from build123d import *

# Parameters (mm, degrees)
BOSS_EXTRUDE1_DEPTH = 1


with BuildPart() as part:
    # Sketch1 → Boss-Extrude1 (new body)
    with BuildSketch(Plane(origin=(0, 0, 0), x_dir=(1, 0, 0), z_dir=(0, 1, 0))):
        with BuildLine():
            Line((-12.25, -13.3), (-12.25, -15))
            Line((-12.25, -15), (12.25, -15))
            Line((12.25, -15), (12.25, -13.3))
            ThreePointArc((12.25, -13.3), (11.50753788, -11.50753788), (13.3, -12.25))
            Line((13.3, -12.25), (15, -12.25))
            Line((15, -12.25), (15, 12.25))
            Line((15, 12.25), (13.3, 12.25))
            ThreePointArc((13.3, 12.25), (11.50753788, 11.50753788), (12.25, 13.3))
            Line((12.25, 13.3), (12.25, 15))
            Line((12.25, 15), (-12.25, 15))
            Line((-12.25, 15), (-12.25, 13.3))
            ThreePointArc((-12.25, 13.3), (-11.50753788, 12.99246212), (-11.2, 12.25))
            ThreePointArc((-11.2, 12.25), (-12.25, 11.2), (-13.3, 12.25))
            Line((-13.3, 12.25), (-15, 12.25))
            Line((-15, 12.25), (-15, -12.25))
            Line((-15, -12.25), (-13.3, -12.25))
            ThreePointArc((-13.3, -12.25), (-12.25, -11.2), (-11.2, -12.25))
            ThreePointArc((-11.2, -12.25), (-11.50753788, -12.99246212), (-12.25, -13.3))
        make_face()
        with BuildLine():
            Line((-15, 12.5), (-15, 12.25))
            Line((-15, 12.25), (-13.3, 12.25))
            ThreePointArc((-13.3, 12.25), (-12.99246212, 12.99246212), (-12.25, 13.3))
            Line((-12.25, 13.3), (-12.25, 15))
            Line((-12.25, 15), (-12.5, 15))
            ThreePointArc((-12.5, 15), (-14.267766953, 14.267766953), (-15, 12.5))
        make_face()
        with BuildLine():
            Line((13.3, 12.25), (15, 12.25))
            Line((15, 12.25), (15, 12.5))
            ThreePointArc((15, 12.5), (14.267766953, 14.267766953), (12.5, 15))
            Line((12.5, 15), (12.25, 15))
            Line((12.25, 15), (12.25, 13.3))
            ThreePointArc((12.25, 13.3), (12.99246212, 12.99246212), (13.3, 12.25))
        make_face()
        with BuildLine():
            Line((12.25, -13.3), (12.25, -15))
            Line((12.25, -15), (12.5, -15))
            ThreePointArc((12.5, -15), (14.267766953, -14.267766953), (15, -12.5))
            Line((15, -12.5), (15, -12.25))
            Line((15, -12.25), (13.3, -12.25))
            ThreePointArc((13.3, -12.25), (12.99246212, -12.99246212), (12.25, -13.3))
        make_face()
        with BuildLine():
            ThreePointArc((-15, -12.5), (-14.267766953, -14.267766953), (-12.5, -15))
            Line((-12.5, -15), (-12.25, -15))
            Line((-12.25, -15), (-12.25, -13.3))
            ThreePointArc((-12.25, -13.3), (-12.99246212, -12.99246212), (-13.3, -12.25))
            Line((-13.3, -12.25), (-15, -12.25))
            Line((-15, -12.25), (-15, -12.5))
        make_face()
    extrude(amount=BOSS_EXTRUDE1_DEPTH)


solid = part.part
Could you check a few things on this model? Use its own coordinates, in mm. Round coordinates to 2 decimals unless told otherwise and drop trailing zeros. Loops run counter-clockwise (first coordinate to the right, second up) from the corner with the lowest first, then second, coordinate; pieces in that order, holes last. Notation, with made-up numbers: (-26.75, 58.5) -> (-7.75, 58.5) arc R25 cw to (-7.75, 88.5) -> close; hole circle Ø3 at (54, -13.75). An arc over 180 degrees is marked (long way). Use CSV: the item, a comma, the result in double quotes.
(1) Will this pin go through, and if not, where does the flat tip stop? pin 1 Ø1.9 at (x, z) = (12.25, -12.25) entering from +Y.
Return value:
pin 1,"passes through"
(2) If I drill on probe 1 along X at (y, z) = (0.35, -12.25); probe 2 along X at (y, z) = (0.8, -11.5), over which ranges is the centre line in solid material (lowest first)? Write a range as [from, to].
Return value:
probe 1,"x = [-15, -13.3], [-11.2, 11.2], [13.3, 15]"
probe 2,"x = [-15, -12.98], [-11.52, 11.52], [12.98, 15]"
(3) Suppose I cut it at A-A on y = 0.15. Write out the boundary of the cut face in (x, z), plus the area to 3 significant figures.
Return value:
outline,"(-15, -12.5) arc R2.5 ccw to (-12.5, -15) -> (12.5, -15) arc R2.5 ccw to (15, -12.5) -> (15, 12.5) arc R2.5 ccw to (12.5, 15) -> (-12.5, 15) arc R2.5 ccw to (-15, 12.5) -> close; hole circle Ø2.1 at (-12.25, -12.25); hole circle Ø2.1 at (-12.25, 12.25); hole circle Ø2.1 at (12.25, -12.25); hole circle Ø2.1 at (12.25, 12.25)"
area,"881 mm²"
